Check sheet for the modelled part. Datum: model origin and axes. Units: mm. A direction names the side the tool comes from. Coordinates: 2 decimals unless noted, no trailing zeros. Write each loop counter-clockwise with the first axis right and the second up, starting at its lowest first coordinate (ties: lowest second). Pieces come first, ordered by that corner, then holes. Notation, with made-up numbers: (44, 52) -> (79, 52) arc R21 cw to (79, 84) -> close; hole circle Ø6 at (-11, 65.25). An arc over 180 degrees is marked (long way). Put each result on its own line as item: value.
```python
from build123d import *

# Parameters (mm, degrees)
HEX_2_DEPTH = 2.286


with BuildPart() as part:
    # BodySke → Base-Revolve (revolve)
    with BuildSketch(Plane.XY, mode=Mode.PRIVATE) as base_revolve_sk:
        Polygon((0, 0), (0, 3.48615), (0.4826, 3.96875), (4.826, 3.96875), (4.826, 2.413), (13.72108, 2.413), (14.351, 1.78308), (14.351, 0), align=None)
    revolve(base_revolve_sk.sketch.rotate(Axis((-31.75, 0, 0), (1, 0, 0)), 90), axis=Axis((-31.75, 0, 0), (1, 0, 0)))  # turned: the seam where the file's is

    # Sketch2 → Hex-PreBroach (revolve, cut)
    with BuildSketch(Plane.XY, mode=Mode.PRIVATE) as hex_prebroach_sk:
        Polygon((0, 1.98501), (2.286, 1.98501), (3.432046058, 0), (0, 0), align=None)
    revolve(hex_prebroach_sk.sketch.rotate(Axis((0, 0, 0), (1, 0, 0)), 90), axis=Axis((0, 0, 0), (1, 0, 0)), mode=Mode.SUBTRACT)  # turned: the seam where the file's is

    # Sketch3 → Hex 2 (cut)
    with BuildSketch(Plane(origin=(0, 0, 0), x_dir=(0, 0.5, 0.866025404), z_dir=(-1, 0, 0))):
        Polygon((1.146046058, 1.98501), (-1.146046058, 1.98501), (-2.292092116, 0), (-1.146046058, -1.98501), (1.146046058, -1.98501), (2.292092116, 0), align=None)
    extrude(amount=-HEX_2_DEPTH, mode=Mode.SUBTRACT)


solid = part.part
```
Q1. Depth check by flat-ended pin: P1, Ø0.5, axis at y = 0.5, z = -1.5, coming from the -X side; P2, Ø1.5, axis at x = 4.5, z = -2.5, coming from the -Y side; P3, Ø1.5, axis at x = 12, y = 1, coming from the -Z side. Enter the tip coordinate at first touch or a pass-through.
Recorded:
P1: stops at x = 2.37
P2: stops at y = -3.56
P3: stops at z = -2.4
Q2. Mould release check, pull along Y, two halves, no side actions. Record for faces 1 (the flat face through (4.826, 2, 2)), 2 (the flat face through (1, 0, 1.985)), 3 (the cylindrical face through (9.336, 1.468, -1.915)): released by +Y, released by -Y, zero draft, split by the parting line, or undercut.
Recorded:
face 1: zero draft
face 2: undercut
face 3: split by the parting line
Q3. Cross-section at A-A (x = 10.25). Record the cut outline in (y, z).
Recorded:
outline: circle Ø4.83 at (0, 0)
Q4. Material ranges on line 1 along Y through (x, z) = (1.75, 0.5); line 2 along X through (y, z) = (-2.5, 0.5); line 3 along Y through (x, z) = (6, 0), recorded low to high.
Recorded:
line 1: y = -3.94 to -2, 2 to 3.94
line 2: x = 0 to 4.83
line 3: y = -2.41 to 2.41
Q5. Tool access check on faces 4 (the flat face through (1, 0, -1.985)), 5 (the cylindrical face through (2.685, 3.874, -0.86)). Record the directions out of +Z, -Z, +X, -X, +Y, -Y that give a thin tool (end or side, any length) a straight path to the whole face; none if there is none.
Recorded:
face 4: -X
face 5: +X, -X
